```python
from build123d import *

# Parameters (mm, degrees)
CROQUIS1_W              = 70
CROQUIS1_H              = 30
CROQUIS1_R              = 3
SALIENTE_EXTRUIR1_DEPTH = 4
CROQUIS3_W              = 70
CROQUIS3_H              = 20
SALIENTE_EXTRUIR2_DEPTH = 4
CROQUIS4_R              = 15
SALIENTE_EXTRUIR3_DEPTH = 80
CROQUIS5_R              = 3
CORTAR_EXTRUIR1_DEPTH   = 4
CROQUIS7_R              = 13.5
CORTAR_EXTRUIR2_DEPTH   = 80
CROQUIS6_R              = 3
CORTAR_EXTRUIR3_DEPTH   = 4
CROQUIS8_W              = 5
CROQUIS8_H              = 15
CORTAR_EXTRUIR4_DEPTH   = 4


with BuildPart() as part:
    # Croquis1 → Saliente-Extruir1 (new body)
    with BuildSketch(Plane.XY):
        Rectangle(CROQUIS1_W, CROQUIS1_H)
        with Locations((0, -5)):
            Circle(CROQUIS1_R, mode=Mode.SUBTRACT)
        with Locations((25, -5)):
            Circle(CROQUIS1_R, mode=Mode.SUBTRACT)
        with Locations((-25, -5)):
            Circle(CROQUIS1_R, mode=Mode.SUBTRACT)
    extrude(amount=SALIENTE_EXTRUIR1_DEPTH)

    # Croquis3 → Saliente-Extruir2 (add)
    with BuildSketch(Plane.XY):
        with Locations((0, 25)):
            Rectangle(CROQUIS3_W, CROQUIS3_H)
    extrude(amount=SALIENTE_EXTRUIR2_DEPTH)

    # Croquis4 → Saliente-Extruir3 (add)
    with BuildSketch(Plane(origin=(0, 0, 0), x_dir=(-1, 0, 0), z_dir=(0, 0, -1))):
        with Locations((0, 15)):
            Circle(CROQUIS4_R)
    extrude(amount=SALIENTE_EXTRUIR3_DEPTH)

    # Croquis5 → Cortar-Extruir1 (cut)
    with BuildSketch(Plane(origin=(0, 0, 0), x_dir=(-1, 0, 0), z_dir=(0, 0, -1))):
        with Locations((-25, 25)):
            Circle(CROQUIS5_R)
        with Locations((25, 25)):
            Circle(CROQUIS5_R)
    extrude(amount=-CORTAR_EXTRUIR1_DEPTH, mode=Mode.SUBTRACT)

    # Croquis7 → Cortar-Extruir2 (cut)
    with BuildSketch(Plane(origin=(0, 0, -80), x_dir=(-1, 0, 0), z_dir=(0, 0, -1))):
        with Locations((0, 15)):
            Circle(CROQUIS7_R)
    extrude(amount=-CORTAR_EXTRUIR2_DEPTH, mode=Mode.SUBTRACT)

    # Croquis6 → Cortar-Extruir3 (cut)
    with BuildSketch(Plane.XY.offset(4)):
        with Locations((0, 15)):
            Circle(CROQUIS6_R)
    extrude(amount=-CORTAR_EXTRUIR3_DEPTH, mode=Mode.SUBTRACT)

    # Croquis8 → Cortar-Extruir4 (cut)
    with BuildSketch(Plane(origin=(0, 0, 0), x_dir=(-1, 0, 0), z_dir=(0, 0, -1))):
        with Locations((-32.5, 27.5)):
            Rectangle(CROQUIS8_W, CROQUIS8_H)
        with Locations((32.5, 27.5)):
            Rectangle(CROQUIS8_W, CROQUIS8_H)
    extrude(amount=-CORTAR_EXTRUIR4_DEPTH, mode=Mode.SUBTRACT)


solid = part.part
```
CAD build for the part. Positions are in the model's coordinates, mm. A direction names the side the tool comes from. Give positions to 0.01 mm unless a question says otherwise; leave off trailing zeros. Order: outer loops, then holes, each group sorted by start corner. A loop starts at its lowest first (then second) coordinate and runs counter-clockwise, first axis right, second up.
(1) Mould opens along Y. For faces 4 (the cylindrical face through (3.252, 0.357, -39.44)), 5 (the cylindrical face through (-27.21, -2.97, 1.97)), 6 (the flat face through (30, 27, 2)), 7 (the flat face through (0, 35, 2)) say: released by +Y, released by -Y, zero draft, split by the parting line, or undercut.
(2) Saw through at B-B, the plane y = -5. Give the cut face in (x, z).
(3) Tool access for faces 1 (the cylindrical face through (1.757, 28.385, -40.56)), 2 (the flat face through (-30, 27, 2)), 3 (the flat face through (33, 20, 2)): list every direction of +Z, -Z, +X, -X, +Y, -Y with a clear straight run to the whole face (end or side of a thin tool).
(4) Saw through at A-A, the plane x = 0. Give the cut face in (y, z), then the cut area to 3 significant figures.
(5) Saw through at D-D, the plane x = -25. Give the cut face in (y, z), then the cut area to 3 significant figures.
(6) Saw through at C-C, the plane y = 25. Give the cut face in (x, z).
(7) Flat gauge pins, fed straight in: pin 1 (6 mm diameter, centred on y = 25, z = -61, fed in from -X); pin 2 (4.5 mm diameter, centred on y = 31, z = 1.5, fed in from -X); pin 3 (2 mm diameter, centred on x = 13, z = -23.5, fed in from -Y); pin 4 (5 mm diameter, centred on x = -25, y = 25, fed in from -Z). Where does each tip first touch, or does it go through?
(8) Drill centre lines: L1, parallel to Y at x = -25, z = 2; L2, parallel to Y at x = 0, z = 0.9; L3, parallel to Y at x = 0, z = -37. Where is each one in solid material? Low to high.
Results found:
1. face 4: split by the parting line
1. face 5: undercut
1. face 6: zero draft
1. face 7: released by +Y
2. outline: (-35, 0) - (-28, 0) - (-28, 4) - (-35, 4) - close; (-22, 0) - (-3, 0) - (-3, 4) - (-22, 4) - close; (3, 0) - (22, 0) - (22, 4) - (3, 4) - close; (28, 0) - (35, 0) - (35, 4) - (28, 4) - close
3. face 1: -Z
3. face 2: +Z, -Z, -X, +Y
3. face 3: +Z, -Z, +X, +Y
4. outline: (-15, 0) - (-8, 0) - (-8, 4) - (-15, 4) - close; (-2, 0) - (0, 0) - (0, -80) - (1.5, -80) - (1.5, 0) - (12, 0) - (12, 4) - (-2, 4) - close; (18, 0) - (28.5, 0) - (28.5, -80) - (30, -80) - (30, 0) - (35, 0) - (35, 4) - (18, 4) - close
4. area: 392 mm2
5. outline: (-15, 0) - (-8, 0) - (-8, 4) - (-15, 4) - close; (-2, 0) - (22, 0) - (22, 4) - (-2, 4) - close; (28, 0) - (35, 0) - (35, 4) - (28, 4) - close
5. area: 152 mm2
6. outline: (-30, 0) - (-28, 0) - (-28, 4) - (-30, 4) - close; (-22, 0) - (-11.18, 0) - (-11.18, -80) - (-9.07, -80) - (-9.07, 0) - (9.07, 0) - (9.07, -80) - (11.18, -80) - (11.18, 0) - (22, 0) - (22, 4) - (-22, 4) - close; (28, 0) - (30, 0) - (30, 4) - (28, 4) - close
7. pin 1: stops at x = -13.27
7. pin 2: stops at x = -30
7. pin 3: stops at y = 6
7. pin 4: passes through
8. L1: y = -15 to -8, -2 to 22, 28 to 35
8. L2: y = -15 to -8, -2 to 12, 18 to 35
8. L3: y = 0 to 1.5, 28.5 to 30
